```python
from build123d import *

# Parameters (mm, degrees)
SKETCH_1_W           = 50
SKETCH_1_H           = 15
SKETCH_1_R           = 1.3
EXTRUDE_1_DEPTH      = 2
SKETCH_2_R           = 2.5
SKETCH_2_R_2         = 1.1
EXTRUDE_2_DEPTH      = 45
EXTRUDE_2_2_DEPTH    = 45
EXTRUDE_START        = 42
EXTRUDE_3_DEPTH      = 5
SKETCH_4_W           = 5
SKETCH_4_H           = 5
EXTRUDE_4_DEPTH      = 40
SKETCH_5_R           = 1.1
CUT_EXTRUDE_1_DEPTH  = 10
EXTRUDE_5_REACH      = 70.307
EXTRUDE_5_END_RADIUS = 2.5
SKETCH_7_W           = 5
SKETCH_7_H           = 10
FILLET_1_R           = 2
EXTRUDE_6_REACH      = 81.107
SKETCH_8_W           = 5
SKETCH_8_H           = 10
FILLET_3_R           = 2


# Read off the part's stored shape, not the designer's step: the extrude step
with BuildPart() as part:
    # Sketch 1 → Extrude 1 (new body)
    with BuildSketch(Plane(origin=(0, 0, 0), x_dir=(1, 0, 0), z_dir=(0, 1, 0))):
        Rectangle(SKETCH_1_W, SKETCH_1_H)
        with Locations(Location((-13.7, 0, 0), (0, 0, 270))):
            Circle(SKETCH_1_R, mode=Mode.SUBTRACT)
        with Locations(Location((13.7, 0, 0), (0, 0, 270))):
            Circle(SKETCH_1_R, mode=Mode.SUBTRACT)
    extrude(amount=EXTRUDE_1_DEPTH)



with BuildPart() as body_2:
    # Sketch 2 → Extrude 2 (new body)
    with BuildSketch(Plane(origin=(0, 2, 0), x_dir=(1, 0, 0), z_dir=(0, 1, 0))):
        with Locations(Location((19.5, 45.3, 0), (0, 0, 90))):
            Circle(SKETCH_2_R)
        with Locations(Location((19.5, 45.3, 0), (0, 0, 90))):
            Circle(SKETCH_2_R_2, mode=Mode.SUBTRACT)
    extrude(amount=EXTRUDE_2_DEPTH)



with BuildPart() as body_3:
    # Sketch 2 → Extrude 2 2 (new body)
    with BuildSketch(Plane(origin=(0, 2, 0), x_dir=(1, 0, 0), z_dir=(0, 1, 0))):
        with Locations(Location((-19.5, 45.3, 0), (0, 0, 90))):
            Circle(SKETCH_2_R)
        with Locations(Location((-19.5, 45.3, 0), (0, 0, 90))):
            Circle(SKETCH_2_R_2, mode=Mode.SUBTRACT)
    extrude(amount=EXTRUDE_2_2_DEPTH)


with BuildPart() as body_2_1:
    add(body_2.part)

    add(body_3.part)  # Extrude 3 merges body 3
    # Extrude 3 outline → Extrude 3 (add)
    with BuildSketch(Plane(origin=(0, 0, 0), x_dir=(1, 0, 0), z_dir=(0, 1, 0)).offset(EXTRUDE_START)):
        with BuildLine():
            Line((-22, 0), (-17, 0))
            Line((-17, 0), (-17, 45.3))
            ThreePointArc((-17, 45.3), (-19.5, 42.8), (-22, 45.3))
            Line((-22, 45.3), (-22, 0))
        make_face()
        with BuildLine():
            Line((17, 45.3), (17, 0))
            Line((17, 0), (22, 0))
            Line((22, 0), (22, 45.3))
            ThreePointArc((22, 45.3), (19.5, 42.8), (17, 45.3))
        make_face()
    extrude(amount=EXTRUDE_3_DEPTH)


with BuildPart() as part_1:
    add(part.part)

    add(body_2_1.part)  # Extrude 4 merges body 2
    # Sketch 4 → Extrude 4 (add)
    with BuildSketch(Plane.XZ.offset(-42)):
        with Locations((19.5, -2.5)):
            Rectangle(SKETCH_4_W, SKETCH_4_H)
        with Locations((-19.5, -2.5)):
            Rectangle(SKETCH_4_W, SKETCH_4_H)
    extrude(amount=EXTRUDE_4_DEPTH)

    # Sketch 5 → Cut-Extrude 1 (cut)
    with BuildSketch(Plane(origin=(0, 47, 0), x_dir=(1, 0, 0), z_dir=(0, 1, 0))):
        with Locations(Location((-19.5, 2.5, 0), (0, 0, 270))):
            Circle(SKETCH_5_R)
        with Locations(Location((19.5, 2.5, 0), (0, 0, 270))):
            Circle(SKETCH_5_R)
    extrude(amount=-CUT_EXTRUDE_1_DEPTH, mode=Mode.SUBTRACT)

    # Extrude 5: up to this cylinder (the profile starts outside it)
    extrude_5_end = Plane(origin=(19.5, 28, -45.3), z_dir=(0, -1, 0)) * Cylinder(EXTRUDE_5_END_RADIUS, 146.614, mode=Mode.PRIVATE)
    # Sketch 7 → Extrude 5 (add, up to the surface)
    with BuildSketch(Plane(origin=(0, 0, -5), x_dir=(-1, 0, 0), z_dir=(0, 0, -1)), mode=Mode.PRIVATE) as extrude_5_sk1:
        with Locations((-19.5, 28)):
            Rectangle(SKETCH_7_W, SKETCH_7_H)
    extrude_5_tool1 = extrude(extrude_5_sk1.sketch, amount=EXTRUDE_5_REACH, mode=Mode.PRIVATE) - extrude_5_end
    add(extrude_5_tool1.solids().sort_by_distance((19.5, 28, -5))[0])

    # Fillet 1
    fillet_1_edges = [part_1.edges().sort_by_distance(p)[0] for p in [
        (25, 1, 7.5),
        (-25, 1, 7.5),
        (-25, 1, -7.5),
        (25, 1, -7.5),
    ]]
    fillet(fillet_1_edges, radius=FILLET_1_R)

    # Sketch 8 → Extrude 6 (add, up to next)
    with BuildSketch(Plane(origin=(-17, 0, 0), x_dir=(0, 0, -1), z_dir=(1, 0, 0)), mode=Mode.PRIVATE) as extrude_6_sk1:
        with Locations((2.5, 28)):
            Rectangle(SKETCH_8_W, SKETCH_8_H)
    extrude_6_tool1 = extrude(extrude_6_sk1.sketch, amount=EXTRUDE_6_REACH, mode=Mode.PRIVATE) - part_1.part
    add(extrude_6_tool1.solids().sort_by_distance((-17, 28, -2.5))[0])

    # Fillet 3
    fillet_3_edges = [part_1.edges().sort_by_distance(p)[0] for p in [
        (-17, 40, 0),
        (17, 40, 0),
        (0, 23, 0),
        (0, 33, 0),
        (17, 12.5, 0),
        (22, 24.5, 0),
        (-22, 24.5, 0),
        (-17, 12.5, 0),
    ]]
    fillet(fillet_3_edges, radius=FILLET_3_R)


solid = part_1.part
```
Can you work these out from the model? Positions are in its coordinate system, mm. A direction names the side the tool comes from. Round coordinates to 2 decimals unless told otherwise and drop trailing zeros. Loops run counter-clockwise (first coordinate to the right, second up) from the corner with the lowest first, then second, coordinate; pieces in that order, holes last. Notation, with made-up numbers: (32.5, 47) -> (38.5, 47) arc R7 ccw to (38.5, 51) -> close; hole circle Ø9 at (45, 32). An arc over 180 degrees is marked (long way). One line per item, written item: value. Start each with the question number.
1. If we section it at B-B, the plane x = -13.7: Write out the boundary of the cut face in (y, z), then the cut area to 3 significant figures.
2. If we section it at C-C, the plane x = -7.5: Write out the boundary of the cut face in (y, z).
3. For faces 4 (the flat face through (17, 13, -4)), 5 (the cylindrical face through (0.27, 32.4, -0.57)), 6 (the cylindrical face through (-20.251, 24.185, -47.685)), which set-ups out of +Z, -Z, +X, -X, +Y, -Y let a thin tool reach every point of the face, with its end or its side?
4. If we section it at A-A, the plane y = 34.5: Write out the boundary of the cut face in (x, z).
5. If I drill on probe 1 along Z at (x, y) = (19.5, 15.5); probe 2 along X at (y, z) = (0.6, 0); probe 3 along X at (y, z) = (17, -45.3), over which ranges is the centre line in solid material (lowest first)?
6. If we section it at D-D, the plane z = -17: Write out the boundary of the cut face in (x, y).
7. If we mould it in two halves opening along X, with no side actions, what happens to faces 1 (the flat face through (-17, 13, -4)), 2 (the cylindrical face through (-21.4, 24.82, -0.57)), 3 (the flat face through (-20, 47, -24))? For each: pulls with the +X half, pulls with the -X half, needs draft (parallel to the pull), parting line crosses it, or undercut.
8. For pin 1 (1 mm diameter, centred on x = 18, y = 37.5, fed in from -Z); pin 2 (5 mm diameter, centred on x = -13, z = -32, fed in from -Y); pin 3 (0.9 mm diameter, centred on y = 7.5, z = -4, fed in from +X); pin 4 (11.5 mm diameter, centred on x = 2.5, y = 29, fed in from -Z), each with a flat end and sliding along its axis, tell me the tip position at first contact or that it passes through.
Calculated:
1. outline: (0, -7.5) -> (2, -7.5) -> (2, -1.3) -> (0, -1.3) -> close; (0, 1.3) -> (2, 1.3) -> (2, 7.5) -> (0, 7.5) -> close; (23, -5) -> (33, -5) -> (33, -2) arc R2 ccw to (31, 0) -> (25, 0) arc R2 ccw to (23, -2) -> close
1. area: 73.1 mm²
2. outline: (0, -7.5) -> (2, -7.5) -> (2, 7.5) -> (0, 7.5) -> close; (23, -5) -> (33, -5) -> (33, -2) arc R2 ccw to (31, 0) -> (25, 0) arc R2 ccw to (23, -2) -> close
3. face 4: +Z, -Z
3. face 5: +Z, +Y
3. face 6: -Y
4. outline: circle Ø5 at (-19.5, -45.3); (-22, -5) -> (-17, -5) -> (-17, -2) arc R2 ccw to (-19, 0) -> (-20, 0) arc R2 ccw to (-22, -2) -> close; circle Ø5 at (19.5, -45.3); (17, -5) -> (22, -5) -> (22, -2) arc R2 ccw to (20, 0) -> (19, 0) arc R2 ccw to (17, -2) -> close; hole circle Ø2.2 at (-19.5, -45.3); hole circle Ø2.2 at (19.5, -45.3)
5. probe 1: z = -47.8 to -46.4, -44.2 to -42.8, -5 to 0
5. probe 2: x = -25 to -15, -12.4 to 12.4, 15 to 25
5. probe 3: x = -22 to -20.6, -18.4 to -17, 17 to 18.4, 20.6 to 22
6. outline: (-22, 42) -> (-17, 42) -> (-17, 47) -> (-22, 47) -> close; (17, 23) -> (22, 23) -> (22, 33) -> (17, 33) -> close; (17, 42) -> (22, 42) -> (22, 47) -> (17, 47) -> close
7. face 1: undercut
7. face 2: pulls with the -X half
7. face 3: needs draft
8. pin 1: stops at z = -47.59
8. pin 2: passes through
8. pin 3: stops at x = 22
8. pin 4: stops at z = -5
